Source: CAD feature listing. Evaluate the final solid. Frame: model axes, mm. A direction names the side the tool comes from. Round coordinates to 2 decimals unless told otherwise and drop trailing zeros. Write each loop counter-clockwise with the first axis right and the second up, starting at its lowest first coordinate (ties: lowest second). Pieces come first, ordered by that corner, then holes.
Autodesk Inventor part; units mm, degrees
ref_plane "YZ Plane" through (0, 0, 0) normal (1, 0, 0) x (0, 1, 0)
ref_plane "XZ Plane" through (0, 0, 0) normal (0, 1, 0) x (-1, 0, 0)
ref_plane "XY Plane" through (0, 0, 0) normal (0, 0, 1) x (1, 0, 0)
sketch "Skizze1" plane through (0, 0, 0) normal (0, 0, 1) x (1, 0, 0)
  line L0 (-7.1596, -18.5) -> (23.8404, -18.5)
  arc A0 (23.8404, -18.5) -> (25.8404, -16.5) centre (23.8404, -16.5) ccw
  line L1 (25.8404, -16.5) -> (25.8404, 16.5)
  arc A1 (25.8404, 16.5) -> (23.8404, 18.5) centre (23.8404, 16.5) ccw
  line L2 (23.8404, 18.5) -> (-23.8404, 18.5)
  arc A2 (-23.8404, 18.5) -> (-25.8404, 16.5) centre (-23.8404, 16.5) ccw
  line L3 (-25.8404, 16.5) -> (-25.8404, -13.1)
  arc A3 (-25.8404, -13.1) -> (-23.8404, -15.1) centre (-23.8404, -13.1) ccw
  line L4 (-23.8404, -15.1) -> (-11.1143, -15.1)
  arc A4 (-9.1369, -16.8) -> (-11.1143, -15.1) centre (-11.1143, -17.1) ccw
  arc A5 (-9.1369, -16.8) -> (-7.1596, -18.5) centre (-7.1596, -16.5) ccw
  line L5 (-24.3404, -13.1) -> (-24.3404, 16.5)
  arc A6 (-23.8404, 17) -> (-24.3404, 16.5) centre (-23.8404, 16.5) ccw
  line L6 (-23.8404, 17) -> (23.8404, 17)
  arc A7 (24.3404, 16.5) -> (23.8404, 17) centre (23.8404, 16.5) ccw
  line L7 (24.3404, 16.5) -> (24.3404, -16.5)
  arc A8 (23.8404, -17) -> (24.3404, -16.5) centre (23.8404, -16.5) ccw
  line L8 (23.8404, -17) -> (-7.1596, -17)
  arc A9 (-7.6539, -16.575) -> (-7.1596, -17) centre (-7.1596, -16.5) ccw
  arc A10 (-7.6539, -16.575) -> (-11.1143, -13.6) centre (-11.1143, -17.1) ccw
  line L9 (-11.1143, -13.6) -> (-23.8404, -13.6)
  arc A11 (-24.3404, -13.1) -> (-23.8404, -13.6) centre (-23.8404, -13.1) ccw
  line L10 (23.8404, 16.7) -> (-23.8404, 16.7)
  arc A12 (-23.8404, 16.7) -> (-24.0404, 16.5) centre (-23.8404, 16.5) ccw
  line L11 (-24.0404, 16.5) -> (-24.0404, -13.1)
  arc A13 (-24.0404, -13.1) -> (-23.8404, -13.3) centre (-23.8404, -13.1) ccw
  line L12 (-23.8404, -13.3) -> (-11.1143, -13.3)
  arc A14 (-7.3573, -16.53) -> (-11.1143, -13.3) centre (-11.1143, -17.1) ccw
  arc A15 (-7.3573, -16.53) -> (-7.1596, -16.7) centre (-7.1596, -16.5) ccw
  line L13 (-7.1596, -16.7) -> (23.8404, -16.7)
  arc A16 (23.8404, -16.7) -> (24.0404, -16.5) centre (23.8404, -16.5) ccw
  line L14 (24.0404, -16.5) -> (24.0404, 16.5)
  arc A17 (24.0404, 16.5) -> (23.8404, 16.7) centre (23.8404, 16.5) ccw
  point P0 (0, 0)
  dimension "d0" = 0.3
extrude "Extrusion1" add sketch "Skizze1" against normal blind 1.5 contours A17 L14 A16 L13 A15 A14 L12 A13 L11 A12 L10
sketch "Skizze2" plane through (0, 0, -1.5) normal (0, 0, -1) x (-1, 0, 0)
  line L0 (6.2404, -13.1) -> (6.2404, 16.5)
  arc A0 (11.1143, -13.3) -> (7.3573, -16.53) centre (11.1143, -17.1) ccw
  arc A1 (7.1596, -16.7) -> (7.3573, -16.53) centre (7.1596, -16.5) ccw
  line L1 (7.1596, -16.7) -> (-23.8404, -16.7)
  arc A2 (-24.0404, -16.5) -> (-23.8404, -16.7) centre (-23.8404, -16.5) ccw
  line L2 (-24.0404, -16.5) -> (-24.0404, 16.5)
  arc A3 (-23.8404, 16.7) -> (-24.0404, 16.5) centre (-23.8404, 16.5) ccw
  line L3 (-23.8404, 16.7) -> (23.8404, 16.7)
  arc A4 (24.0404, 16.5) -> (23.8404, 16.7) centre (23.8404, 16.5) ccw
  line L4 (24.0404, 16.5) -> (24.0404, -13.1)
  arc A5 (23.8404, -13.3) -> (24.0404, -13.1) centre (23.8404, -13.1) ccw
  line L5 (23.8404, -13.3) -> (11.1143, -13.3)
  line L6 (5.2404, -37.9441) -> (-28.2922, -37.9441)
  line L7 (-28.2922, -37.9441) -> (-28.2922, 30.637)
  line L8 (-28.2922, 30.637) -> (5.2404, 30.637)
  line L9 (5.2404, 30.637) -> (5.2404, -37.9441)
  point P0 (0, 0)
  point P1 (5.2404, -16.7)
  point P2 (5.2404, 16.7)
  dimension "d3" = 1
extrude "Extrusion2" add sketch "Skizze2" along normal blind 3 contours L1 A2 L2 A3 L3 L9
sketch "Skizze3" plane through (-7.1596, -16.7, 0) normal (0, -1, 0) x (1, 0, 0)
  circle A0 centre (28, -3) radius 2
  circle A1 centre (4, -3) radius 2
  circle A2 centre (28, -3) radius 0.9
  circle A3 centre (4, -3) radius 0.9
  point P0 (7.1596, 0)
  dimension "d6" = 1.8
  dimension "d7" = 1.8
extrude "Extrusion3" cut sketch "Skizze3" against normal through all contours A2 | A3
chamfer "Fase1" distance 0.5 angle 45 4 edges at (-4.0596, 16.7, -3) (19.9404, 16.7, -3) (19.9404, -16.7, -3) (-4.0596, -16.7, -3)
properties part number "Boden"
1) Contact query for flat-ended pins moving along their axis: P1, Ø2, axis at x = 20.84, z = -3, coming from the +Y side; P2, Ø2.5, axis at x = -3.16, z = -3, coming from the +Y side; P3, Ø15, axis at x = -15, y = 6.5, coming from the -Z side. Output: stop coordinate, or through.
Taken from the geometry:
P1: stops at y = 16.3
P2: stops at y = 16.55
P3: stops at z = -1.5
2) Section query B-B on y = -1. Return the cut outline in (x, z), then the cut area to 3 significant figures.
Taken from the geometry:
outline: (-24.04, -1.5) - (-5.24, -1.5) - (-5.24, -4.5) - (24.04, -4.5) - (24.04, 0) - (-24.04, 0) - close; hole circle Ø1.8 at (-3.16, -3); hole circle Ø1.8 at (20.84, -3)
area: 155 mm2
3) Reachability of faces 1 (the face through (-5.24, 0, -3)), 2 (the face through (-18, -13.3, -1)), 3 (the face through (24.04, 0, -2)) from +Z, -Z, +X, -X, +Y, -Y: full face, straight path, thin tool, end or side. Return the list, or none.
Taken from the geometry:
face 1: -Z, -X, +Y, -Y
face 2: +Z, -Z, -X, -Y
face 3: +Z, -Z, +X, +Y, -Y
4) Section query D-D on x = -19. Return the cut outline in (y, z).
Taken from the geometry:
outline: (-13.3, -1.5) - (16.7, -1.5) - (16.7, 0) - (-13.3, 0) - close
5) Section query A-A on z = -3. Return the cut outline in (x, y).
Taken from the geometry:
outline: (-5.24, -16.7) - (-4.56, -16.7) - (-4.06, -16.2) - (-4.06, 16.2) - (-4.56, 16.7) - (-5.24, 16.7) - close; (-2.26, -16.2) - (-1.76, -16.7) - (19.44, -16.7) - (19.94, -16.2) - (19.94, 16.2) - (19.44, 16.7) - (-1.76, 16.7) - (-2.26, 16.2) - close; (21.74, -16.2) - (22.24, -16.7) - (23.84, -16.7) arc R0.2 ccw to (24.04, -16.5) - (24.04, 16.5) arc R0.2 ccw to (23.84, 16.7) - (22.24, 16.7) - (21.74, 16.2) - close
6) Material intervals for line 1 (X direction, y = -10, z = -3.75); line 2 (X direction, y = -12, z = -3.5); line 3 (Y direction, x = -18, z = -1.4), sorted ascending.
Taken from the geometry:
line 1: x = -5.24 to -3.66, -2.66 to 20.34, 21.34 to 24.04
line 2: x = -5.24 to -3.91, -2.41 to 20.09, 21.59 to 24.04
line 3: y = -13.3 to 16.7
7) Pull-direction query (X, two-part tool) for faces 4 (the face through (-8.61, -14.24, -0.74)), 5 (the face through (0, 0, 0)), 6 (the face through (21.672, -0.227, -3.345)), 7 (the face through (-3.35, -0.23, -3.88)); classes: released by +X, released by -X, zero draft, split by the parting line, or undercut.
Taken from the geometry:
face 4: released by -X
face 5: zero draft
face 6: undercut
face 7: undercut
8) Section query C-C on z = -0.85. Return the cut outline in (x, y), then the cut area to 3 significant figures.
Taken from the geometry:
outline: (-24.04, -13.1) arc R0.2 ccw to (-23.84, -13.3) - (-11.11, -13.3) arc R3.8 cw to (-7.36, -16.53) arc R0.2 ccw to (-7.16, -16.7) - (23.84, -16.7) arc R0.2 ccw to (24.04, -16.5) - (24.04, 16.5) arc R0.2 ccw to (23.84, 16.7) - (-23.84, 16.7) arc R0.2 ccw to (-24.04, 16.5) - close
area: 1,550 mm2
